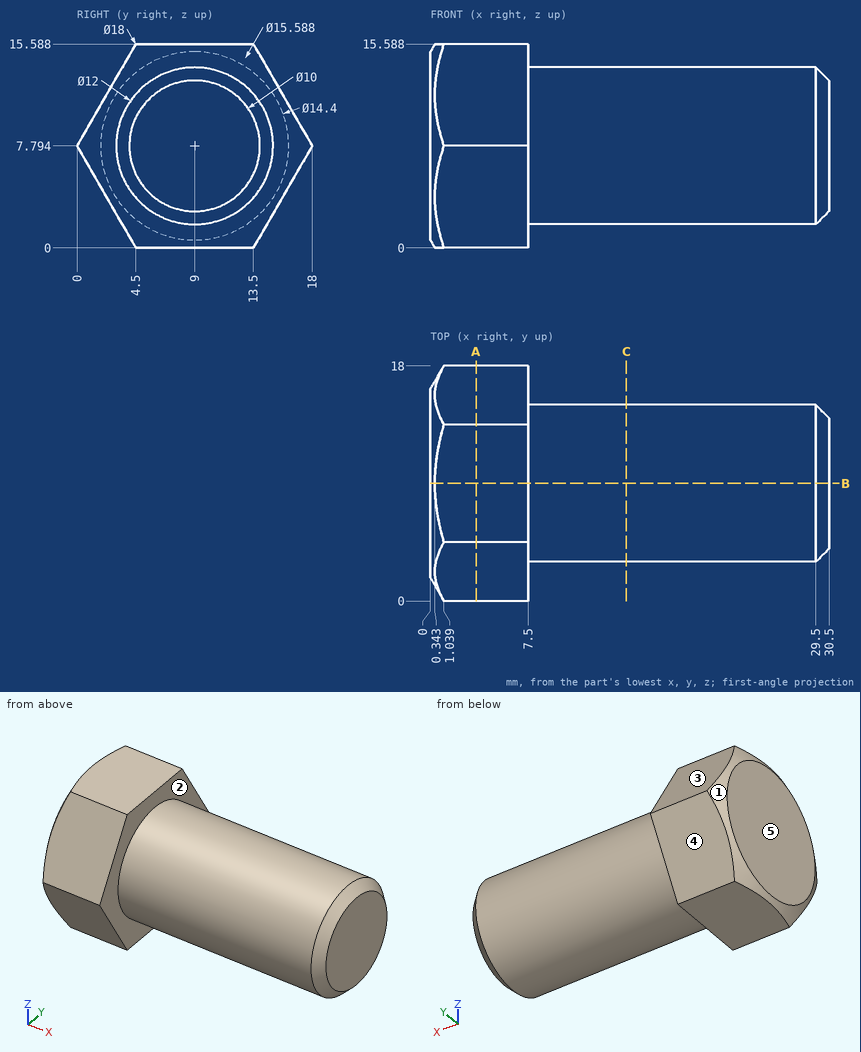
Answer from the drawing. Dimensions are ordinates in mm from the lowest x, y and z of the part. A direction names the side the tool comes from. Coordinates: 2 decimals unless noted, no trailing zeros. Order: outer loops, then holes, each group sorted by start corner. A loop starts at its lowest first (then second) coordinate and runs counter-clockwise, first axis right, second up. Notation, with made-up numbers: (53.5, -34) -> (59.5, -34) arc R20 cw to (59.5, -4) -> close; hole circle Ø1 at (-24, -0.5). An arc over 180 degrees is marked (long way). Answer as a JSON object with one key per item and string values.
1) Each of these flat-tipped pins is pushed along its axis until it touches: pin 1 (6 mm diameter, centred on x = 11.5, z = 3, fed in from +Y) (1 decimal); pin 2 (8 mm diameter, centred on x = 14, y = 8, fed in from +Z); pin 3 (5 mm diameter, centred on x = 14.5, z = 7.5, fed in from +Y). Where does it stop, or does it pass through?
Model answer:
{"pin 1": "stops at y = 14.7", "pin 2": "stops at z = 13.79", "pin 3": "stops at y = 15"}
2) The mould has two halves that part along Z. Classify the marked faces 3, 4 and 5: released by +Z, released by -Z, zero draft, split by the parting line, or undercut.
Model answer:
{"face 3": "released by +Z", "face 4": "released by -Z", "face 5": "zero draft"}
3) A cutting plane is placed at B-B, the plane y = 9. Determine the outline of the cut face in (x, z) (1 decimal), plus the area to 3 significant figures.
Model answer:
{"outline": "(0, 0.6) -> (0.3, 0) -> (7.5, 0) -> (7.5, 1.8) -> (29.5, 1.8) -> (30.5, 2.8) -> (30.5, 12.8) -> (29.5, 13.8) -> (7.5, 13.8) -> (7.5, 15.6) -> (0.3, 15.6) -> (0, 15) -> close", "area": "392 mm²"}
4) A cutting plane is placed at C-C, the plane x = 15. Determine the outline of the cut face in (y, z) (1 decimal).
Model answer:
{"outline": "circle Ø12 at (9, 7.8)"}
5) A cutting plane is placed at A-A, the plane x = 3.5. Determine the outline of the cut face in (y, z) (1 decimal), plus the area to 3 significant figures.
Model answer:
{"outline": "(0, 7.8) -> (4.5, 0) -> (13.5, 0) -> (18, 7.8) -> (13.5, 15.6) -> (4.5, 15.6) -> close", "area": "210 mm²"}
6) A tool of negligible diameter and unlimited length cuts with its end or side. For the marked faces 1 and 2, from which of +Z, -Z, +X, -X, +Y, -Y can it reach the whole face along a straight path? Write none if from no direction.
Model answer:
{"face 1": "-X", "face 2": "+X"}
7) Consider line 1 along X through (y, z) = (14.5, 3.75); line 2 along Y through (x, z) = (21, 7.5); line 3 along Z through (x, y) = (18.5, 8.75). Determine where each line is inside the solid, lowest interval first. Write a range as from..to.
Model answer:
{"line 1": "x = 0..7.5", "line 2": "y = 3.01..14.99", "line 3": "z = 1.8..13.79"}
